Geometry: final body of the model. Coordinates: model frame, mm. Give positions to 0.01 mm unless a question says otherwise; leave off trailing zeros. Loops run counter-clockwise (first coordinate to the right, second up) from the corner with the lowest first, then second, coordinate; pieces in that order, holes last.
from build123d import *

# Parameters (mm, degrees)
F0_W     = 170
F0_H     = 230
F1_DEPTH = 5
F2_R     = 3
F3_DEPTH = 5
F4_R     = 2.5
F5_DEPTH = 5
F6_R     = 3
F7_DEPTH = 5
F8_R     = 3
F9_DEPTH = 5


with BuildPart() as f1:
    # F0 (on Front) → F1 (new body)
    with BuildSketch(Plane.XZ):
        Rectangle(F0_W, F0_H)
    extrude(amount=F1_DEPTH)

    # F2 (on face) → F3 (cut)
    with BuildSketch(Plane.XZ.offset(5)):
        with Locations((-57.5, 108.5)):
            Circle(F2_R)
        with Locations((-22.5, 108.5)):
            Circle(F2_R)
        with Locations((-57.5, 73.5)):
            Circle(F2_R)
        with Locations((-22.5, 73.5)):
            Circle(F2_R)
        with Locations((22.5, 108.5)):
            Circle(F2_R)
        with Locations((22.5, 73.5)):
            Circle(F2_R)
        with Locations((57.5, 73.5)):
            Circle(F2_R)
        with Locations((57.5, 108.5)):
            Circle(F2_R)
        with Locations((57.5, -1.5)):
            Circle(F2_R)
        with Locations((22.5, -1.5)):
            Circle(F2_R)
        with Locations((22.353769, -36.5)):
            Circle(F2_R)
        with Locations((57.5, -36.5)):
            Circle(F2_R)
        with Locations((-22.5, -1.5)):
            Circle(F2_R)
        with Locations((-57.5, -1.5)):
            Circle(F2_R)
        with Locations((-22.353769, -36.5)):
            Circle(F2_R)
        with Locations((-57.5, -36.5)):
            Circle(F2_R)
    extrude(amount=-F3_DEPTH, mode=Mode.SUBTRACT)

    # F4 (on face) → F5 (cut)
    with BuildSketch(Plane.XZ.offset(5)):
        with Locations((-12, 56)):
            Circle(F4_R)
        with Locations((-12, 16)):
            Circle(F4_R)
        with Locations((12, 56)):
            Circle(F4_R)
        with Locations((12, 16)):
            Circle(F4_R)
    extrude(amount=-F5_DEPTH, mode=Mode.SUBTRACT)

    # F6 (on face) → F7 (cut)
    with BuildSketch(Plane.XZ.offset(5)):
        with Locations((37.5, 53.5)):
            Circle(F6_R)
        with BuildLine():
            ThreePointArc((69.5, 53.5), (72.5, 50.5), (75.5, 53.5))
            ThreePointArc((75.5, 53.5), (72.5, 56.5), (69.5, 53.5))
        make_face()
        with Locations((37.5, 18.5)):
            Circle(F6_R)
        with Locations((72.5, 18.5)):
            Circle(F6_R)
        with Locations((-37.5, 53.5)):
            Circle(F6_R)
        with Locations((-72.5, 53.5)):
            Circle(F6_R)
        with Locations((-37.5, 18.5)):
            Circle(F6_R)
        with Locations((-72.5, 18.5)):
            Circle(F6_R)
    extrude(amount=-F7_DEPTH, mode=Mode.SUBTRACT)

    # F8 (on face) → F9 (cut)
    with BuildSketch(Plane.XZ.offset(5)):
        with Locations((-37.5, -56.5)):
            Circle(F8_R)
        with Locations((-72.5, -56.5)):
            Circle(F8_R)
        with Locations((-37.5, -91.5)):
            Circle(F8_R)
        with Locations((-72.5, -91.5)):
            Circle(F8_R)
        with Locations((37.5, -56.5)):
            Circle(F8_R)
        with Locations((72.5, -56.5)):
            Circle(F8_R)
        with Locations((37.5, -91.5)):
            Circle(F8_R)
        with Locations((72.5, -91.5)):
            Circle(F8_R)
    extrude(amount=-F9_DEPTH, mode=Mode.SUBTRACT)


solid = f1.part
Item 1: Pin query (flat end, axial travel): pin 1 (5 mm diameter, centred on x = 37.5, z = 18.5, fed in from -Y). Return the tip coordinate at first contact, or that it passes through.
Values follow:
pin 1: passes through
Item 2: Section query A-A on z = -1.5. Return loops of the section in (x, y), plus the area to 3 significant figures.
Values follow:
outline: (-85, -5) - (-60.5, -5) - (-60.5, 0) - (-85, 0) - close; (-54.5, -5) - (-25.5, -5) - (-25.5, 0) - (-54.5, 0) - close; (-19.5, -5) - (19.5, -5) - (19.5, 0) - (-19.5, 0) - close; (25.5, -5) - (54.5, -5) - (54.5, 0) - (25.5, 0) - close; (60.5, -5) - (85, -5) - (85, 0) - (60.5, 0) - close
area: 730 mm2
Item 3: Ray query, probe 1 along Z at (x, y) = (-57.5, -3.1); probe 2 along Z at (x, y) = (-37.5, -1.35); probe 3 along X at (y, z) = (-3.95, -89.5). Return the intervals inside material, ascending.
Values follow:
probe 1: z = -115 to -39.5, -33.5 to -4.5, 1.5 to 70.5, 76.5 to 105.5, 111.5 to 115
probe 2: z = -115 to -94.5, -88.5 to -59.5, -53.5 to 15.5, 21.5 to 50.5, 56.5 to 115
probe 3: x = -85 to -74.74, -70.26 to -39.74, -35.26 to 35.26, 39.74 to 70.26, 74.74 to 85
Item 4: Section query B-B on y = -3.95. Give the number of separate pieces and of enclosed holes in the cut face, plus the area to 3 significant figures.
Values follow:
separate pieces: 1
enclosed holes: 36
area: 38,100 mm2
Item 5: Draft query along X for faces 1 (the face through (72.109, -2.535, 56.474)), 2 (the face through (85, -2, -2)), 3 (the face through (-1, -2, -115)). Return one class per face: +X half, -X half, draft (parallel to the pull), parting line (faces both ways), or undercut.
Values follow:
face 1: undercut
face 2: +X half
face 3: draft
